Read the model definition and answer for the solid it produces. Units are mm, in the model's axes. Coordinates: 2 decimals unless noted, no trailing zeros. Write each loop counter-clockwise with the first axis right and the second up, starting at its lowest first coordinate (ties: lowest second). Pieces come first, ordered by that corner, then holes. Notation, with made-up numbers: (-9, 54.5) -> (25, 54.5) arc R17 ccw to (25, 62.5) -> close; hole circle Ø5 at (24, 57). An arc over 180 degrees is marked (long way). Answer as a JSON object with one key per item and string values. Group by question number.
(1) Find section D-D (y = -0.1). Count the separate pieces of the cut face and the enclosed holes in it, then the cut area to 3 significant figures.
(2) For a pull along Z with two mould halves and no side action, classify faces 1 (the face through (-41.774, -0.028, 30.923)), 2 (the face through (-86.37, -0.03, -17.78)), 3 (the face through (-5, -2, -1)) as +Z half, -Z half, draft (parallel to the pull), parting line (faces both ways), or undercut.
(3) Find section C-C (z = 34). Give the vertices of the cut face in (x, y).
(4) Flat-ended cylindrical pins translate along their axes: P1, Ø2, axis at x = 33, y = 1, coming from the -Z side; P2, Ø2, axis at y = -0.5, z = 58.5, coming from the -X side; P3, Ø1.5, axis at y = 1, z = -37, coming from the +X side. Find the tip coordinate at first contact, or state that the pin passes through.
(5) Straight lines are drawn through the part: L1, parallel to X at y = -0.9, z = 20; L2, parallel to Z at x = -22, y = -0.65; L3, parallel to Z at x = 39, y = -0.65. For each, find the intervals that lie inside material, in ascending order.
(6) Find section A-A (z = -20). Give the vertices of the cut face in (x, y), then the cut area to 3 significant figures.
(7) Find section B-B (x = 60). Give the vertices of the cut face in (y, z).
from build123d import *

# Parameters (mm, degrees)
EXTRUDE_2426_DEPTH          = 2
CUT_EXTRUDE_2700_DEPTH      = 184.109257002
CUT_EXTRUDE_2700_DEPTH_BACK = 184.109257002
SKETCH_5_R                  = 92
SKETCH_5_R_2                = 82
VV_DEPTH                    = 121.533854246
VV_DEPTH_BACK               = 121.533854246
CUT_EXTRUDE_7_DEPTH         = 121.533854246
CUT_EXTRUDE_7_DEPTH_BACK    = 121.533854246
SKETCH_10_R                 = 2
CUT_EXTRUDE_8_DEPTH         = 121.533854246
CUT_EXTRUDE_8_DEPTH_BACK    = 121.533854246
SKETCH_17_R                 = 2
CUT_EXTRUDE_9_DEPTH         = 121.533854246
CUT_EXTRUDE_9_DEPTH_BACK    = 121.533854246
SKETCH_6_R                  = 2


with BuildPart() as part:
    # 草图1 → Extrude 2426 (new, symmetric)
    with BuildSketch(Plane(origin=(0, 0, 0), x_dir=(1, 0, 0), z_dir=(0, 1, 0))):
        Polygon((-150, -85), (-150, 85), (-110, 85), (-69, 85), (-62, 85), (-25, 105), (-2, 105), (30, 105), (56.423376881, 85), (67.423376881, 85), (108.643784617, 85), (108.643784617, 70), (123.423376881, 70), (138, 40), (150, 40), (150, -40), (138, -40), (123.423376881, -70), (108.643784617, -70), (108.643784617, -85), (67.423376881, -85), (56.423376881, -85), (30, -105), (-2, -105), (-25, -105), (-62, -85), (-69, -85), (-110, -85), align=None)
    extrude(amount=EXTRUDE_2426_DEPTH, both=True)

    # 草图5 → Cut-Extrude 2700 (cut, two sides: drawn at the far end of the back side and taken through both)
    with BuildSketch(Plane(origin=(0, 0, 0), x_dir=(1, 0, 0), z_dir=(0, 1, 0)).offset(-CUT_EXTRUDE_2700_DEPTH_BACK)):
        with Locations((-6.31992991, 0)):
            Circle(SKETCH_5_R)
        with Locations(Location((-6.31992991, 0, 0), (0, 0, 270))):
            Circle(SKETCH_5_R_2, mode=Mode.SUBTRACT)
    extrude(amount=CUT_EXTRUDE_2700_DEPTH + CUT_EXTRUDE_2700_DEPTH_BACK, mode=Mode.SUBTRACT)


with BuildPart() as body_2:
    # of the pieces the cut leaves, the one that is kept (cut_extrude_2700_keep)
    add(part.part.solids().sort_by_distance((-6.31992991, -2, 82))[0])

    # 草图11 → vv (cut, two sides: drawn at the far end of the back side and taken through both)
    with BuildSketch(Plane(origin=(0, 0, 0), x_dir=(1, 0, 0), z_dir=(0, 1, 0)).offset(-VV_DEPTH_BACK)):
        Polygon((6.325153319, 64.535132696), (-23.677770795, 55.665092595), (-23.677770795, 47.002272942), (6.325153319, 32.096278657), (6.325153319, 39.061910109), (-17.161984245, 50.730744019), (6.325153319, 57.674462279), align=None)
        Polygon((4.981591187, -30.190121431), (-25.021332927, -39.060161532), (-25.021332927, -47.722981185), (4.981591187, -62.62897547), (4.981591187, -55.663344018), (-18.505546377, -43.994510108), (4.981591187, -37.050791848), align=None)
    extrude(amount=VV_DEPTH + VV_DEPTH_BACK, mode=Mode.SUBTRACT)

    # 草图10 → 切除-拉伸7 (cut, two sides: drawn at the far end of the back side and taken through both)
    with BuildSketch(Plane(origin=(0, 0, 0), x_dir=(1, 0, 0), z_dir=(0, 1, 0)).offset(-CUT_EXTRUDE_7_DEPTH_BACK)):
        with Locations((-130, 65)):
            Circle(SKETCH_10_R)
        with Locations((-130, -65)):
            Circle(SKETCH_10_R)
        with Locations((115, 55)):
            Circle(SKETCH_10_R)
        with Locations((115, -55)):
            Circle(SKETCH_10_R)
        with Locations(Location((-60, 20, 0), (0, 0, 270))):
            Circle(SKETCH_10_R)
        with Locations(Location((-60, -20, 0), (0, 0, 270))):
            Circle(SKETCH_10_R)
        with Locations(Location((60, 20, 0), (0, 0, 270))):
            Circle(SKETCH_10_R)
        with Locations(Location((60, -20, 0), (0, 0, 270))):
            Circle(SKETCH_10_R)
    extrude(amount=CUT_EXTRUDE_7_DEPTH + CUT_EXTRUDE_7_DEPTH_BACK, mode=Mode.SUBTRACT)

    # 草图17 → 切除-拉伸8 (cut, two sides: drawn at the far end of the back side and taken through both)
    with BuildSketch(Plane(origin=(0, 0, 0), x_dir=(1, 0, 0), z_dir=(0, 1, 0)).offset(-CUT_EXTRUDE_8_DEPTH_BACK)):
        with Locations(Location((-40, 30, 0), (0, 0, 270))):
            Circle(SKETCH_17_R)
        with Locations(Location((40, 30, 0), (0, 0, 270))):
            Circle(SKETCH_17_R)
        with Locations(Location((-40, -30, 0), (0, 0, 270))):
            Circle(SKETCH_17_R)
        with Locations(Location((40, -30, 0), (0, 0, 270))):
            Circle(SKETCH_17_R)
    extrude(amount=CUT_EXTRUDE_8_DEPTH + CUT_EXTRUDE_8_DEPTH_BACK, mode=Mode.SUBTRACT)

    # 草图6 → 切除-拉伸9 (cut, two sides: drawn at the far end of the back side and taken through both)
    with BuildSketch(Plane(origin=(0, 0, 0), x_dir=(1, 0, 0), z_dir=(0, 1, 0)).offset(-CUT_EXTRUDE_9_DEPTH_BACK)):
        with Locations(Location((21.774981178, -12.387805022, 0), (0, 0, 270))):
            Circle(SKETCH_6_R)
        with Locations(Location((-9.265018822, 10.892194978, 0), (0, 0, 270))):
            Circle(SKETCH_6_R)
        with Locations(Location((-9.265018822, -12.387805022, 0), (0, 0, 270))):
            Circle(SKETCH_6_R)
        with Locations(Location((6.254981178, -0.747805022, 0), (0, 0, 270))):
            Circle(SKETCH_6_R)
        with Locations(Location((21.774981178, 10.892194978, 0), (0, 0, 270))):
            Circle(SKETCH_6_R)
    extrude(amount=CUT_EXTRUDE_9_DEPTH + CUT_EXTRUDE_9_DEPTH_BACK, mode=Mode.SUBTRACT)


solid = body_2.part
Results below:
{
 "1": {"separate pieces": "1", "enclosed holes": "15", "area": "20,200 mm2"},
 "2": {"face 1": "undercut", "face 2": "parting line", "face 3": "draft"},
 "3": {"outline": "(-80.94, -2) -> (-7.91, -2) -> (-7.91, 2) -> (-80.94, 2) -> close; (4.98, -2) -> (68.3, -2) -> (68.3, 2) -> (4.98, 2) -> close"},
 "4": {"P1": "stops at z = -72.5", "P2": "stops at x = -64.78", "P3": "stops at x = 67.23"},
 "5": {"L1": "x = -85.84 to -62, -58 to 58, 62 to 73.2", "L2": "z = -80.49 to -56.16, -46.17 to 38.17, 49.22 to 80.49", "L3": "z = -68.34 to -31.73, -28.27 to 28.27, 31.73 to 68.34"},
 "6": {"outline": "(-85.84, -2) -> (-62, -2) -> (-62, 2) -> (-85.84, 2) -> close; (-58, -2) -> (58, -2) -> (58, 2) -> (-58, 2) -> close; (62, -2) -> (73.2, -2) -> (73.2, 2) -> (62, 2) -> close", "area": "604 mm2"},
 "7": {"outline": "(-2, -48.23) -> (2, -48.23) -> (2, -22) -> (-2, -22) -> close; (-2, -18) -> (2, -18) -> (2, 18) -> (-2, 18) -> close; (-2, 22) -> (2, 22) -> (2, 48.23) -> (-2, 48.23) -> close"}
}
